from build123d import *

# Parameters (mm, degrees)
SKETCH_3_R      = 2
SKETCH_3_R_2    = 1.5
EXTRUDE_1_DEPTH = 2


with BuildPart() as part:
    # 草图3 → 凸台-拉伸1 (new body)
    with BuildSketch(Plane.XY):
        with BuildLine():
            Line((-46.5, 63), (-37.576612526, 61.656694359))
            ThreePointArc((-37.576612526, 61.656694359), (-11.38853896, 19.746708007), (34.06116735, 39.152540881))
            Line((34.06116735, 39.152540881), (41, 39.152540881))
            Line((41, 39.152540881), (45, 31.317051182))
            Line((45, 31.317051182), (45, 25.109783315))
            Line((45, 25.109783315), (30.045120352, -16.062768097))
            Line((30.045120352, -16.062768097), (19.571056376, -21.44452782))
            ThreePointArc((19.571056376, -21.44452782), (16.636857193, -21.33673956), (15.2, -18.776156704))
            Line((15.2, -18.776156704), (15.2, 8.509783315))
            Line((15.2, 8.509783315), (0, 8.509783315))
            Line((0, 8.509783315), (-15.2, 8.509783315))
            Line((-15.2, 8.509783315), (-15.2, -18.776156704))
            ThreePointArc((-15.2, -18.776156704), (-16.636857193, -21.33673956), (-19.571056376, -21.44452782))
            Line((-19.571056376, -21.44452782), (-30.045120352, -16.062768097))
            Line((-30.045120352, -16.062768097), (-46.5, 28.773494756))
            Line((-46.5, 28.773494756), (-46.5, 63))
        make_face()
        with Locations((0, 13.5)):
            Circle(SKETCH_3_R, mode=Mode.SUBTRACT)
        with Locations((-42.5, 56)):
            Circle(SKETCH_3_R, mode=Mode.SUBTRACT)
        with Locations((30.0520382, 25.9479618)):
            Circle(SKETCH_3_R, mode=Mode.SUBTRACT)
        with Locations((-30.045120352, 25.954879648)):
            Circle(SKETCH_3_R, mode=Mode.SUBTRACT)
        with Locations((-25, -1.990216685)):
            Circle(SKETCH_3_R_2, mode=Mode.SUBTRACT)
        with Locations((-25, 13.509783315)):
            Circle(SKETCH_3_R_2, mode=Mode.SUBTRACT)
        with Locations(Location((25, 13.509783315, 0), (0, 0, 180))):
            Circle(SKETCH_3_R_2, mode=Mode.SUBTRACT)
        with Locations(Location((25, -1.990216685, 0), (0, 0, 180))):
            Circle(SKETCH_3_R_2, mode=Mode.SUBTRACT)
    extrude(amount=EXTRUDE_1_DEPTH)


solid = part.part
Design review of the part built by this model. Coordinates are the model's own, in mm. A direction names the side the tool comes from. Coordinates: 2 decimals unless noted, no trailing zeros. Loops run counter-clockwise (first coordinate to the right, second up) from the corner with the lowest first, then second, coordinate; pieces in that order, holes last. Notation, with made-up numbers: (57, 68) -> (88, 68) arc R8 ccw to (88, 76) -> close; hole circle Ø2 at (-39.75, -31.5). An arc over 180 degrees is marked (long way). Use a Markdown table: item, result. Add a question column.
Item 1: We need section B-B, the plane y = 56. Write out the cut boundary in (x, z), and give its area (3 significant figures).
Item 2: We need section C-C, the plane z = 0.75. Count the separate pieces of the cut face and the enclosed holes in it, and give its area (4 significant figures).
Item 3: Wall thickness on L1, parallel to X at y = 13, z = 0.1; L2, parallel to Y at x = 25, z = 0.7; L3, parallel to X at y = 27, z = 1.3: over which ranges is each line inside the solid? List them lowest first. Write a range as from..to.
Item 4: Clearance check with flat-ended pins moving along their axes: P1, Ø0.6, axis at x = 2, z = 0.5, coming from the -Y side; P2, Ø0.6, axis at y = -5, z = 1, coming from the +X side. State where each tip first meets the part, or that it passes through.
Item 5: We need section D-D, the plane x = 25. Write out the cut boundary in (y, z), and give its area (3 significant figures).
Item 6: The part is to be moulded in two halves that separate along X. For faces 3 (the flat face through (45, 28, 1)), 4 (the cylindrical face through (-26.5, 13.58, 0.99)), 5 (the cylindrical face through (-16.6, -21.314, 0.986)), 6 (the flat face through (-46.5, 46, 1)), say which applies: +X half, -X half, draft (parallel to the pull), parting line (faces both ways), or undercut.
Item 7: Machinability: for faces 1 (the flat face through (-38.157, 6.042, 0.986)), 2 (the flat face through (-15.2, -5, 1)), which of the approach directions +Z, -Z, +X, -X, +Y, -Y give a long, thin tool a straight path to every point of the face, cutting with its end or side? Answer none if there is none.
Item 8: We need section A-A, the plane x = 0. Write out the cut boundary in (y, z), and give its area (3 significant figures).
Numbers:
| question | item | result |
|---|---|---|
| 1 | outline | (-46.5, 0) -> (-44.5, 0) -> (-44.5, 2) -> (-46.5, 2) -> close; (-40.5, 0) -> (-38, 0) -> (-38, 2) -> (-40.5, 2) -> close |
| 1 | area | 9.00 mm^2 |
| 2 | separate pieces | 1 |
| 2 | enclosed holes | 8 |
| 2 | area | 2,825 mm^2 |
| 3 | L1 | x = -40.71..-26.41, -23.59..-1.94, 1.94..23.59, 26.41..40.6 |
| 3 | L2 | y = -18.66..-3.49, -0.49..12.01, 15.01..27.38 |
| 3 | L3 | x = -45.85..-31.75, -28.34..-24.56, 24.56..28.35, 31.75..45 |
| 4 | P1 | stops at y = 8.51 |
| 4 | P2 | stops at x = 34.17 |
| 5 | outline | (-18.66, 0) -> (-3.49, 0) -> (-3.49, 2) -> (-18.66, 2) -> close; (-0.49, 0) -> (12.01, 0) -> (12.01, 2) -> (-0.49, 2) -> close; (15.01, 0) -> (27.38, 0) -> (27.38, 2) -> (15.01, 2) -> close |
| 5 | area | 80.1 mm^2 |
| 6 | face 3 | +X half |
| 6 | face 4 | undercut |
| 6 | face 5 | undercut |
| 6 | face 6 | -X half |
| 7 | face 1 | +Z, -Z, -X, -Y |
| 7 | face 2 | +Z, -Z, -Y |
| 8 | outline | (8.51, 0) -> (11.5, 0) -> (11.5, 2) -> (8.51, 2) -> close; (15.5, 0) -> (18, 0) -> (18, 2) -> (15.5, 2) -> close |
| 8 | area | 11.0 mm^2 |
